from build123d import *

# Parameters (mm, degrees)
BOSS_EXTRUDE1_DEPTH = 2.54
SKETCH2_R           = 0.6
CUT_EXTRUDE1_DEPTH  = 92.616219088
BOSS_EXTRUDE2_DEPTH = 1.27
CUT_EXTRUDE2_DEPTH  = 1.27
SKETCH5_R           = 2.499995
CUT_EXTRUDE3_DEPTH  = 92.616219088
SKETCH6_R           = 9.525
CUT_EXTRUDE4_DEPTH  = 10.16


with BuildPart() as part:
    # Sketch1 → Boss-Extrude1 (new body)
    with BuildSketch(Plane(origin=(0, 0, 0), x_dir=(1, 0, 0), z_dir=(0, 1, 0))):
        with BuildLine():
            Line((63.5, 50.8), (-63.5, 50.8))
            ThreePointArc((-63.5, 50.8), (-72.480256121, 47.080256121), (-76.2, 38.1))
            Line((-76.2, 38.1), (-76.2, -38.1))
            ThreePointArc((-76.2, -38.1), (-72.480256121, -47.080256121), (-63.5, -50.8))
            Line((-63.5, -50.8), (63.5, -50.8))
            ThreePointArc((63.5, -50.8), (72.480256121, -47.080256121), (76.2, -38.1))
            Line((76.2, -38.1), (76.2, 38.1))
            ThreePointArc((76.2, 38.1), (72.480256121, 47.080256121), (63.5, 50.8))
        make_face()
    extrude(amount=BOSS_EXTRUDE1_DEPTH)

    # Sketch2 → Cut-Extrude1 (cut, through all)
    with BuildSketch(Plane(origin=(0, 2.54, 0), x_dir=(1, 0, 0), z_dir=(0, 1, 0))):
        with Locations(Location((-71.628, 46.228, 0), (0, 0, 270))):
            Circle(SKETCH2_R)
        with Locations(Location((-71.628, -46.228, 0), (0, 0, 270))):
            Circle(SKETCH2_R)
        with Locations(Location((71.628, -46.228, 0), (0, 0, 270))):
            Circle(SKETCH2_R)
        with Locations(Location((71.628, 46.228, 0), (0, 0, 270))):
            Circle(SKETCH2_R)
    extrude(amount=-CUT_EXTRUDE1_DEPTH, mode=Mode.SUBTRACT)

    # Sketch3 → Boss-Extrude2 (add)
    with BuildSketch(Plane(origin=(0, 2.54, 0), x_dir=(1, 0, 0), z_dir=(0, 1, 0))):
        with BuildLine():
            Line((63.5, 44.45), (-5.08, 44.45))
            ThreePointArc((-5.08, 44.45), (-7.774076836, 43.334076836), (-8.89, 40.64))
            Line((-8.89, 40.64), (-8.89, -40.64))
            ThreePointArc((-8.89, -40.64), (-7.774076836, -43.334076836), (-5.08, -44.45))
            Line((-5.08, -44.45), (63.5, -44.45))
            ThreePointArc((63.5, -44.45), (66.194076836, -43.334076836), (67.31, -40.64))
            Line((67.31, -40.64), (67.31, 40.64))
            ThreePointArc((67.31, 40.64), (66.194076836, 43.334076836), (63.5, 44.45))
        make_face()
    extrude(amount=BOSS_EXTRUDE2_DEPTH)

    # Sketch4 → Cut-Extrude2 (cut)
    with BuildSketch(Plane(origin=(0, 3.81, 0), x_dir=(1, 0, 0), z_dir=(0, 1, 0))):
        with BuildLine():
            Line((-5.08, 41.91), (63.5, 41.91))
            ThreePointArc((63.5, 41.91), (64.398025612, 41.538025612), (64.77, 40.64))
            Line((64.77, 40.64), (64.77, -40.64))
            ThreePointArc((64.77, -40.64), (64.398025612, -41.538025612), (63.5, -41.91))
            Line((63.5, -41.91), (-5.08, -41.91))
            ThreePointArc((-5.08, -41.91), (-5.978025612, -41.538025612), (-6.35, -40.64))
            Line((-6.35, -40.64), (-6.35, 40.64))
            ThreePointArc((-6.35, 40.64), (-5.978025612, 41.538025612), (-5.08, 41.91))
        make_face()
    extrude(amount=-CUT_EXTRUDE2_DEPTH, mode=Mode.SUBTRACT)

    # Sketch5 → Cut-Extrude3 (cut, through all)
    with BuildSketch(Plane(origin=(0, 2.54, 0), x_dir=(1, 0, 0), z_dir=(0, 1, 0))):
        with Locations(Location((11.43, 20.955, 0), (0, 0, 270))):
            Circle(SKETCH5_R)
        with Locations(Location((46.99, 20.955, 0), (0, 0, 270))):
            Circle(SKETCH5_R)
        with Locations(Location((11.43, -20.955, 0), (0, 0, 270))):
            Circle(SKETCH5_R)
        with Locations(Location((46.99, -20.955, 0), (0, 0, 270))):
            Circle(SKETCH5_R)
    extrude(amount=-CUT_EXTRUDE3_DEPTH, mode=Mode.SUBTRACT)

    # Sketch6 → Cut-Extrude4 (cut)
    with BuildSketch(Plane(origin=(0, 2.54, 0), x_dir=(1, 0, 0), z_dir=(0, 1, 0))):
        with Locations(Location((-38.1, 0, 0), (0, 0, 270))):
            Circle(SKETCH6_R)
    extrude(amount=-CUT_EXTRUDE4_DEPTH, mode=Mode.SUBTRACT)


solid = part.part
Could you check a few things on this model? Use its own coordinates, in mm. A direction names the side the tool comes from. Coordinates: 2 decimals unless noted, no trailing zeros. Write each loop counter-clockwise with the first axis right and the second up, starting at its lowest first coordinate (ties: lowest second). Pieces come first, ordered by that corner, then holes. Notation, with made-up numbers: M 80.25,4.25 L 118.25,4.25 A24 cw 118.25,43.25 Z; hole C -33,64 d3. An arc over 180 degrees is marked long. One line per question, with ' | ' between items.
1) For pin 1 Ø1.6 at (x, z) = (71.628, 46.228) entering from +Y; pin 2 Ø4 at (x, z) = (46.99, 20.955) entering from -Y; pin 3 Ø1.4 at (x, y) = (17, 3.5) entering from -Z; pin 4 Ø0.6 at (x, y) = (34, 3) entering from +Z, each with a flat end and sliding along its axis, tell me the tip position at first contact or that it passes through.
Checks:
pin 1: y = 2.54 | pin 2: through | pin 3: z = -44.45 | pin 4: z = 44.45
2) Imagine slicing it at D-D, the plane y = 0.75. Give the number of separate pieces and of enclosed holes in the cut face, and give its area (3 significant figures).
Checks:
separate pieces: 1 | enclosed holes: 9 | area: 15,000 mm²
3) Imagine slicing it at A-A, the plane x = 11.43. Write out the boundary of the cut face in (y, z) (3 decimals), and give its area (3 significant figures).
Checks:
outline: M 0,-50.8 L 2.54,-50.8 L 2.54,-44.45 L 3.81,-44.45 L 3.81,-41.91 L 2.54,-41.91 L 2.54,-23.455 L 0,-23.455 Z; M 0,-18.455 L 2.54,-18.455 L 2.54,18.455 L 0,18.455 Z; M 0,23.455 L 2.54,23.455 L 2.54,41.91 L 3.81,41.91 L 3.81,44.45 L 2.54,44.45 L 2.54,50.8 L 0,50.8 Z | area: 239 mm²
4) For faces 5 (the face through (-7.744, 3.166, -43.364)), 6 (the face through (66.164, 3.166, 43.364)), 7 (the face through (-7.804, 3.166, 43.304)), which set-ups out of +Z, -Z, +X, -X, +Y, -Y let a thin tool reach every point of the face, with its end or its side?
Checks:
face 5: -Z, -X, +Y | face 6: +Z, +X, +Y | face 7: +Z, -X, +Y
5) I need wall thicknesses on probe 1 along X at (y, z) = (2.6, -29.5); probe 2 along Z at (x, y) = (11.5, 3.2); probe 3 along Y at (x, z) = (-21, -40.5). Which ranges of each line are inside material? Lowest first, please. Write a range as [from, to].
Checks:
probe 1: [-8.89, -6.35], [64.77, 67.31] | probe 2: [-44.45, -41.91], [41.91, 44.45] | probe 3: [0, 2.54]
6) Imagine slicing it at B-B, the plane z = 0. Write out the boundary of the cut face in (x, y) (3 decimals).
Checks:
outline: M -76.2,0 L -47.625,0 L -47.625,2.54 L -76.2,2.54 Z; M -28.575,0 L 76.2,0 L 76.2,2.54 L 67.31,2.54 L 67.31,3.81 L 64.77,3.81 L 64.77,2.54 L -6.35,2.54 L -6.35,3.81 L -8.89,3.81 L -8.89,2.54 L -28.575,2.54 Z
7) If we mould it in two halves opening along X, with no side actions, what happens to faces 1 (the face through (49.47, 1.29, 20.63)), 2 (the face through (-1, 0, -1)), 3 (the face through (30, 2.54, -1)), 4 (the face through (66.224, 3.166, -43.304))? For each: released by +X, released by -X, zero draft, split by the parting line, or undercut.
Checks:
face 1: undercut | face 2: zero draft | face 3: undercut | face 4: released by +X
8) Imagine slicing it at C-C, the plane x = -38.1. Write out the boundary of the cut face in (y, z) (3 decimals).
Checks:
outline: M 0,-50.8 L 2.54,-50.8 L 2.54,-9.525 L 0,-9.525 Z; M 0,9.525 L 2.54,9.525 L 2.54,50.8 L 0,50.8 Z
